Part model, mm, in its own coordinate system. Face numbers are marked on the shaded views. A direction names the side the tool comes from. Round coordinates to 2 decimals unless told otherwise and drop trailing zeros. Order: outer loops, then holes, each group sorted by start corner. A loop starts at its lowest first (then second) coordinate and runs counter-clockwise, first axis right, second up. Notation, with made-up numbers: M 55,68.5 L 78,68.5 A10 ccw 78,72.5 Z; hole C -13.75,-14.5 d10. An arc over 180 degrees is marked long. One line per question, with ' | ' between items.
from build123d import *

# Parameters (mm, degrees)
F0_W     = 61.481372
F0_H     = 9.264317
F1_DEPTH = 25.4
F2_W     = 11.790948
F2_H     = 22.739682
F3_DEPTH = 6.35
F4_W     = 36.215054
F4_H     = 19.90229
F5_DEPTH = 38.602317


with BuildPart() as f1:
    # F0 (on Top) → F1 (new body)
    with BuildSketch(Plane.XY):
        with Locations((0, 33.969158)):
            Rectangle(F0_W, F0_H)
    extrude(amount=F1_DEPTH)

    # F2 (on Top) → F3 (join)
    with BuildSketch(Plane.XY):
        with Locations((-24.564476, 18.528631)):
            Rectangle(F2_W, F2_H)
        with Locations((24.564476, 18.528631)):
            Rectangle(F2_W, F2_H)
    extrude(amount=F3_DEPTH)

    # F4 (on Front) → F5 (cut, through all)
    with BuildSketch(Plane.XZ):
        with Locations((-1e-06, 9.951145)):
            Rectangle(F4_W, F4_H)
    extrude(amount=-F5_DEPTH, mode=Mode.SUBTRACT)


solid = f1.part
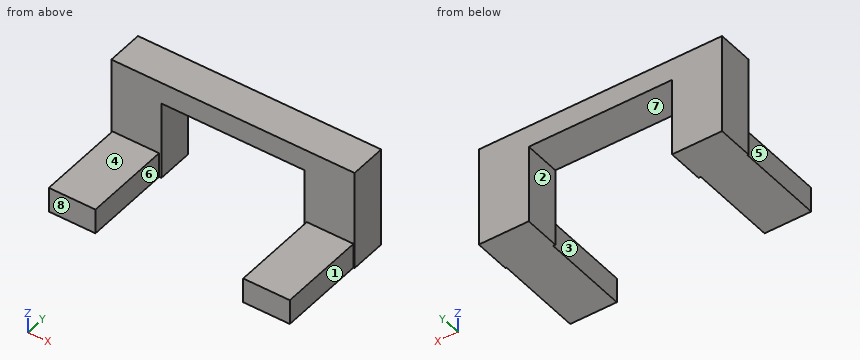
1) Saw through at C-C (y = 36). List the corners of the cut face in (x, z), plus the area to 3 significant figures.
The answers:
outline: M -30.74,0 L -18.11,0 L -18.11,19.9 L 18.11,19.9 L 18.11,0 L 30.74,0 L 30.74,25.4 L -30.74,25.4 Z | area: 841 mm²
2) Probe line 1 (X direction, y = 26.5, z = 2); line 2 (X direction, y = 30, z = 19.75); line 3 (Z direction, x = -19, y = 11.5). List the from-to ranges inside material, lowest first. Write a range as [from, to].
The answers:
line 1: x = [-30.46, -18.67], [18.67, 30.46] | line 2: x = [-30.74, -18.11], [18.11, 30.74] | line 3: z = [0, 6.35]
3) Two-plate mould, pull along X, no slides. Class the marked faces 5, 6, 7 and 8: released by +X, released by -X, zero draft, split by the parting line, or undercut.
The answers:
face 5: released by -X | face 6: undercut | face 7: undercut | face 8: zero draft
4) Which spindle directions (+Z, -Z, +X, -X, +Y, -Y) get a long thin tool onto all of the face, cutting with end or side? Do the marked faces 1, 2, 3 and 4. Say none if no direction does.
The answers:
face 1: +Z, -Z, +X, -Y | face 2: -Z, +Y, -Y | face 3: +Z, -Z, -Y | face 4: +Z, +X, -X, -Y
5) Saw through at B-B (y = 17.5). List the corners of the cut face in (x, z), plus the area to 3 significant figures.
The answers:
outline: M -30.46,0 L -18.67,0 L -18.67,6.35 L -30.46,6.35 Z; M 18.67,0 L 30.46,0 L 30.46,6.35 L 18.67,6.35 Z | area: 150 mm²
6) Saw through at A-A (z = 5.5). List the corners of the cut face in (x, y).
The answers:
outline: M -30.74,29.34 L -30.46,29.34 L -30.46,7.16 L -18.67,7.16 L -18.67,29.34 L -18.11,29.34 L -18.11,38.6 L -30.74,38.6 Z; M 18.11,29.34 L 18.67,29.34 L 18.67,7.16 L 30.46,7.16 L 30.46,29.34 L 30.74,29.34 L 30.74,38.6 L 18.11,38.6 Z
7) Saw through at D-D (z = 9.75). List the corners of the cut face in (x, y).
The answers:
outline: M -30.74,29.34 L -18.11,29.34 L -18.11,38.6 L -30.74,38.6 Z; M 18.11,29.34 L 30.74,29.34 L 30.74,38.6 L 18.11,38.6 Z
8) Drop flat-ended pins along their axis: pin 1 (7 mm diameter, centred on y = 13, z = 3, fed in from +X); pin 2 (13 mm diameter, centred on x = 24, y = 18, fed in from +Z); pin 3 (1.9 mm diameter, centred on y = 16.5, z = 3.5, fed in from -X). Give the stop position or say it passes through.
The answers:
pin 1: stops at x = 30.46 | pin 2: stops at z = 6.35 | pin 3: stops at x = -30.46
